Verification items for the finished model (mm, model axes). Face numbers are marked on the shaded views. A direction names the side the tool comes from. Coordinates: 2 decimals unless noted, no trailing zeros. Write each loop counter-clockwise with the first axis right and the second up, starting at its lowest first coordinate (ties: lowest second). Pieces come first, ordered by that corner, then holes. Notation, with made-up numbers: (22, 13.25) -> (51, 13.25) arc R17 cw to (51, 43.25) -> close; hole circle Ø7 at (60, 5.5). An arc over 180 degrees is marked (long way). Use CSV: the item, a comma, the result in double quotes.
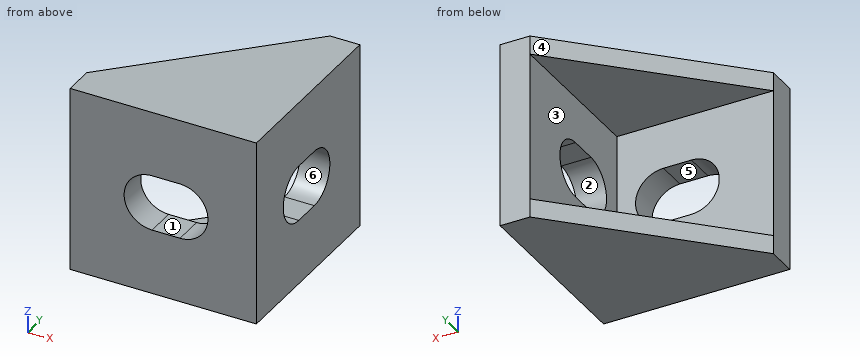
Autodesk Inventor part; units mm, degrees
ref_plane "YZ Plane" through (0, 0, 0) normal (1, 0, 0) x (0, 1, 0)
ref_plane "XZ Plane" through (0, 0, 0) normal (0, 1, 0) x (-1, 0, 0)
ref_plane "XY Plane" through (0, 0, 0) normal (0, 0, 1) x (1, 0, 0)
sketch "Sketch1" plane through (0, 0, 0) normal (0, 1, 0) x (-1, 0, 0)
  line L0 (0, 0) -> (20, 0)
  line L1 (20, 0) -> (20, -20)
  line L2 (20, -20) -> (0, -20)
  line L3 (0, -20) -> (0, 0)
  dimension "d0" = 20
  dimension "d1" = 20
extrude "Extrusion1" add sketch "Sketch1" along normal blind 20
sketch "Sketch2" plane through (-20, 0, 0) normal (0, 0, 1) x (1, 0, 0)
  line L0 (20, 0) -> (0, 0)
  line L1 (20, 0) -> (20, 20)
  line L2 (20, 20) -> (0, 20)
  line L3 (0, 20) -> (16.8, 20)
  line L4 (0, 0) -> (0, 20)
  line L5 (1.6773, 3.2839) -> (0, 3.1156)
  line L6 (0, 20) -> (0, 3.2)
  line L7 (16.8, 20) -> (0, 3.2)
  dimension "d6" = 16.8
  dimension "d9" = 16.8
extrude "Extrusion3" cut sketch "Sketch2" against normal blind 20 contours L7 L4 L2
sketch "Sketch3" plane through (0, 20, 0) normal (0, 1, 0) x (1, 0, 0)
  line L0 (0, 18) -> (-20, 18)
  line L1 (-20, 18) -> (-20, 2)
  line L2 (-20, 2) -> (0, 2)
  line L3 (0, 2) -> (0, 18)
  line L4 (-20, 20) -> (-3.2, 20)
  line L5 (-4, 18) -> (12, 18) construction
  line L6 (0, 18) -> (0, 2)
  line L7 (-3.2, 18) -> (-3.2, 2)
  point P0 (-20, 10)
  dimension "d12" = 16
  dimension "d13" = 2
extrude "Extrusion4" cut sketch "Sketch3" against normal blind 16.8 contours L7 L2 L1 L0
sketch "Sketch4" plane through (0, 3.2, 0) normal (0, 1, 0) x (1, 0, 0)
  line L0 (-14.2, 13) -> (-5.2, 13)
  line L1 (-5.2, 13) -> (-5.2, 7)
  line L2 (-5.2, 7) -> (-14.2, 7)
  line L3 (-14.2, 7) -> (-14.2, 13)
  line L4 (-3.2, 18) -> (-3.2, 2)
  arc A0 (-8.2, 7) -> (-8.2, 13) centre (-8.2, 10) ccw
  line L5 (-18, 13.026) -> (-18, 7.026)
  line L6 (-20, 2) -> (-20, 18)
  ellipse E0 centre (-14.2, 10) end of major axis (-18, 10) minor radius 3 (-14.2, 13) -> (-14.2, 7) ccw
  arc A1 (-11.2, 13) -> (-11.2, 7) centre (-11.2, 10) ccw
  line L7 (-5.2, 10) -> (-18, 10)
  line L8 (-20, 18) -> (-3.2, 18)
  point P0 (0, 0)
  dimension "d18" = 6
  dimension "d19" = 9
  dimension "d20" = 2
  dimension "d21" = 6
  dimension "d22" = 2
  dimension "d40" = 8
extrude "Extrusion5" cut sketch "Sketch4" against normal blind 16.8 contours L0 A0 L7 A1 | L7 A0 L2 A1
sketch "Sketch8" plane through (-3.2, 0.3648, -21.4635) normal (-1, 0, 0) x (0, -1, 0)
  line L0 (-13.8352, 14.4635) -> (-4.8352, 14.4635)
  line L1 (-4.8352, 14.4635) -> (-4.8352, 8.4635)
  line L2 (-4.8352, 8.4635) -> (-13.8352, 8.4635)
  line L3 (-13.8352, 8.4635) -> (-13.8352, 14.4635)
  line L4 (-2.8352, 18) -> (-2.8352, 2)
  arc A0 (-7.8352, 8.4635) -> (-7.8352, 14.4635) centre (-7.8352, 11.4635) ccw
  line L5 (-18, 13.026) -> (-18, 7.026)
  line L6 (-20, 2) -> (-20, 18)
  ellipse E0 centre (-13.8352, 11.4635) end of major axis (-18, 11.4635) minor radius 3 (-13.8352, 14.4635) -> (-13.8352, 8.4635) ccw
  arc A1 (-10.8352, 14.4635) -> (-10.8352, 8.4635) centre (-10.8352, 11.4635) ccw
  line L7 (-4.8352, 11.4635) -> (-18, 11.4635)
  line L8 (-2.8352, 19.4635) -> (-2.8352, 3.4635)
  line L9 (-19.6352, 19.4635) -> (-2.8352, 19.4635)
  point P0 (0, 0)
  dimension "d34" = 6
  dimension "d33" = 9
  dimension "d32" = 2
  dimension "d31" = 6
  dimension "d30" = 2
  dimension "d38" = 0
  dimension "d39" = 5
extrude "Extrusion7" cut sketch "Sketch8" against normal blind 16.8 contours L0 A0 L7 A1 | L7 A0 L2 A1
properties part number "Al_Bracket"
1) Cross-section at A-A (z = -10). Record the boundary of the cut face in (x, y).
Return value:
outline,"(-20, 0) -> (-14.2, 0) -> (-14.2, 3.2) -> (-20, 3.2) -> close; (-5.2, 0) -> (0, 0) -> (0, 5.2) -> (-3.2, 5.2) -> (-3.2, 3.2) -> (-5.2, 3.2) -> close; (-3.2, 14.2) -> (0, 14.2) -> (0, 20) -> (-3.2, 20) -> close"
2) Scan lines: L1, parallel to Z at x = -6, y = 9.75; L2, parallel to Y at x = -7.5, z = -17.75; L3, parallel to Z at x = -3, y = 10.25. Record each from-to range of solid material in increasing order.
Return value:
L1,"-20 to -18, -2 to 0"
L2,"0 to 3.2"
L3,"-20 to -13, -7 to 0"
3) Mould release check, pull along Y, two halves, no side actions. Record for the marked faces 4, 5 and 6: released by +Y, released by -Y, zero draft, split by the parting line, or undercut.
Return value:
face 4,"released by +Y"
face 5,"zero draft"
face 6,"undercut"
4) Set-up check for the marked faces 1, 2 and 3: record each of +Z, -Z, +X, -X, +Y, -Y from which the full face is reachable in a straight line by a thin tool's end or side.
Return value:
face 1,"+Y, -Y"
face 2,"+X, -X"
face 3,"-X, +Y"
5) Cross-section at C-C (x = -1.75). Record the boundary of the cut face in (y, z), plus the area to 3 significant figures.
Return value:
outline,"(0, -20) -> (20, -20) -> (20, 0) -> (0, 0) -> close; hole (8.2, -13) -> (11.2, -13) arc R3 ccw to (11.2, -7) -> (8.2, -7) arc R3 ccw to start"
area,"354 mm2"
6) Cross-section at B-B (y = 1.75). Record the boundary of the cut face in (x, z).
Return value:
outline,"(-20, -20) -> (0, -20) -> (0, 0) -> (-20, 0) -> close; hole (-11.2, -13) -> (-8.2, -13) arc R3 ccw to (-8.2, -7) -> (-11.2, -7) arc R3 ccw to start"
7) Cross-section at D-D (x = -5.5). Record the boundary of the cut face in (y, z), plus the area to 3 significant figures.
Return value:
outline,"(0, -20) -> (17.7, -20) -> (17.7, -18) -> (3.2, -18) -> (3.2, -11.31) -> (0, -11.31) -> close; (0, -8.69) -> (3.2, -8.69) -> (3.2, -2) -> (17.7, -2) -> (17.7, 0) -> (0, 0) -> close"
area,"114 mm2"
8) Gauge pin test, flat ends, axial feed: pin 1 (1.5 mm diameter, centred on x = -8.5, y = 9.5, fed in from +Z); pin 2 (3 mm diameter, centred on x = -8, z = -11, fed in from +Y); pin 3 (3 mm diameter, centred on y = 17.5, z = -13, fed in from -X); pin 4 (1.5 mm diameter, centred on x = -5, z = -16, fed in from +Y). Record the tip position at first contact, or that the pin passes through.
Return value:
pin 1,"z = 0"
pin 2,"through"
pin 3,"x = -3.2"
pin 4,"y = 3.2"
